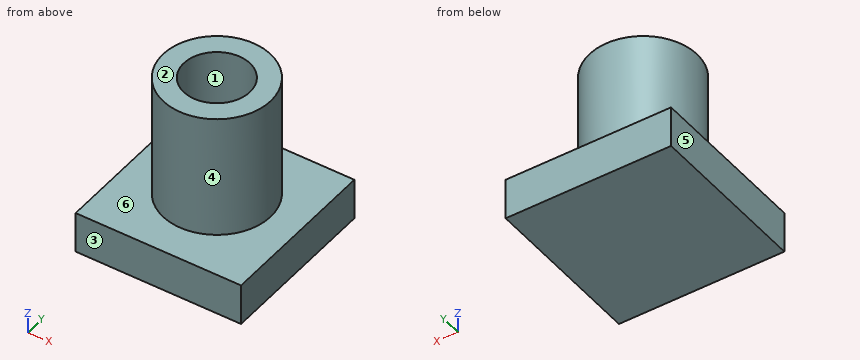
from build123d import *

# Parameters (mm, degrees)
F0_W     = 25.4
F0_H     = 25.4
F1_DEPTH = 6.35
F2_R     = 8.255
F2_R_2   = 5.08
F3_DEPTH = 25.4


with BuildPart() as f1:
    # F0 (on Top) → F1 (new body)
    with BuildSketch(Plane.XY):
        with Locations((-25.977274, 37.378409)):
            Rectangle(F0_W, F0_H)
    extrude(amount=F1_DEPTH)

    # F2 (on Top) → F3 (join)
    with BuildSketch(Plane.XY):
        with Locations((-26.134709, 38.018856)):
            Circle(F2_R)
        with Locations((-26.134709, 38.018856)):
            Circle(F2_R_2, mode=Mode.SUBTRACT)
    extrude(amount=F3_DEPTH)


solid = f1.part
Here's how the part is built. I have some questions about the finished solid (model axes, mm). Face numbers are marked on the shaded views. A direction names the side the tool comes from. Coordinates: 2 decimals unless noted, no trailing zeros. Order: outer loops, then holes, each group sorted by start corner. A loop starts at its lowest first (then second) coordinate and runs counter-clockwise, first axis right, second up.
Item 1: If we section it at C-C on z = 19: List the corners of the cut face in (x, y) for me (3 decimals), plus the area to 3 significant figures.
Result sheet:
outline: circle Ø16.51 at (-26.135, 38.019); hole circle Ø10.16 at (-26.135, 38.019)
area: 133 mm2
Item 2: If we section it at D-D on y = 36.5: List the corners of the cut face in (x, z) for me, plus the area to 3 significant figures.
Result sheet:
outline: (-38.68, 0) - (-13.28, 0) - (-13.28, 6.35) - (-18.02, 6.35) - (-18.02, 25.4) - (-21.29, 25.4) - (-21.29, 6.35) - (-30.98, 6.35) - (-30.98, 25.4) - (-34.25, 25.4) - (-34.25, 6.35) - (-38.68, 6.35) - close
area: 286 mm2
Item 3: I need wall thicknesses on line 1 (Z direction, x = -31, y = 45); line 2 (Y direction, x = -22.25, z = 12.25); line 3 (Y direction, x = -21.5, z = 18). Which ranges of each line are inside material? Lowest first, please.
Result sheet:
line 1: z = 0 to 6.35
line 2: y = 30.74 to 34.75, 41.29 to 45.3
line 3: y = 31.19 to 35.94, 40.1 to 44.85
Item 4: For the marked faces 5 and 6, which set-ups out of +Z, -Z, +X, -X, +Y, -Y let a thin tool reach every point of the face, with its end or its side?
Result sheet:
face 5: +Z, -Z, -X, +Y, -Y
face 6: +Z
Item 5: If we section it at B-B on y = 44.75: List the corners of the cut face in (x, z) for me.
Result sheet:
outline: (-38.68, 0) - (-13.28, 0) - (-13.28, 6.35) - (-21.36, 6.35) - (-21.36, 25.4) - (-30.91, 25.4) - (-30.91, 6.35) - (-38.68, 6.35) - close
Item 6: For P1, Ø4, axis at y = 37.5, z = 13, coming from the +X side; P2, Ø2, axis at x = -28, z = 12, coming from the -Y side; P3, Ø3, axis at x = -25.5, y = 38, coming from the +Z side, each with a flat end and sliding along its axis, tell me the tip position at first contact or that it passes through.
Result sheet:
P1: stops at x = -17.88
P2: stops at y = 29.81
P3: stops at z = 6.35
Item 7: If we section it at A-A on x = -18.5: List the corners of the cut face in (y, z) for me.
Result sheet:
outline: (24.68, 0) - (50.08, 0) - (50.08, 6.35) - (41.16, 6.35) - (41.16, 25.4) - (34.88, 25.4) - (34.88, 6.35) - (24.68, 6.35) - close
Item 8: If we mould it in two halves opening along Y, with no side actions, what happens to the marked faces 1, 2, 3 and 4? For each: +Y half, -Y half, draft (parallel to the pull), parting line (faces both ways), or undercut.
Result sheet:
face 1: undercut
face 2: draft
face 3: -Y half
face 4: parting line
